Here's how the part is built. I have some questions about the finished solid (model axes, mm). Face numbers are marked on the shaded views. A direction names the side the tool comes from. Round coordinates to 2 decimals unless told otherwise and drop trailing zeros. Write each loop counter-clockwise with the first axis right and the second up, starting at its lowest first coordinate (ties: lowest second). Pieces come first, ordered by that corner, then holes. Notation, with made-up numbers: M 28.25,89 L 67.25,89 A25 ccw 67.25,113 Z; hole C 69.5,32 d8. An arc over 180 degrees is marked long. Use one line per item in the form item = value. Start each with the question number.
Q1. I want a section at A-A on y = -18.5. List the corners of the cut face in (x, z) for me, and give its area (3 significant figures).
Q2. For the marked faces 1, 2 and 3, which set-ups out of +Z, -Z, +X, -X, +Y, -Y let a thin tool reach every point of the face, with its end or its side?
Q3. I want a section at C-C on x = 33. List the corners of the cut face in (y, z) for me, and give its area (3 significant figures).
Q4. I'm going to push flat-ended pins straight in: pin 1 Ø20 at (x, y) = (-30.5, -21.5) entering from +Z; pin 2 Ø7.5 at (y, z) = (-14, 7.5) entering from +X; pin 3 Ø17.5 at (y, z) = (-27.5, -1.5) entering from -X; pin 4 Ø7 at (x, y) = (45, -28.5) entering from +Z. Where does each tip first touch, or does it pass through?
Q5. I want a section at B-B on z = 4. List the corners of the cut face in (x, y) for me.
Q6. I need wall thicknesses on line 1 along X through (y, z) = (-26, -1); line 2 along Z through (x, y) = (49.5, -29.5); line 3 along Z through (x, y) = (-27.5, -25). Which ranges of each line are inside material? Lowest first, please. Write a range as from..to.
```python
from build123d import *

# Parameters (mm, degrees)
F0_W     = 100.000054
F0_H     = 59.99988
F1_DEPTH = 39.99992
F2_W     = 23.5305579296
F2_H     = 25.0000008
F2_W_2   = 25.0000008
F2_H_2   = 34.99993
F3_DEPTH = 40.00092


with BuildPart() as f1:
    # F0 (on Front) → F1 (new body)
    with BuildSketch(Plane.XZ):
        with Locations((3.9102658629, -8.0880385926)):
            Rectangle(F0_W, F0_H)
    extrude(amount=F1_DEPTH)

    # F2 (on face) → F3 (cut, through all)
    with BuildSketch(Plane.XZ.offset(39.99992)):
        with Locations((42.1450138982, 9.4119010074)):
            Rectangle(F2_W, F2_H)
        with Locations((-33.5897607371, 4.4119364074)):
            Rectangle(F2_W_2, F2_H_2)
    extrude(amount=-F3_DEPTH, mode=Mode.SUBTRACT)


solid = f1.part
```
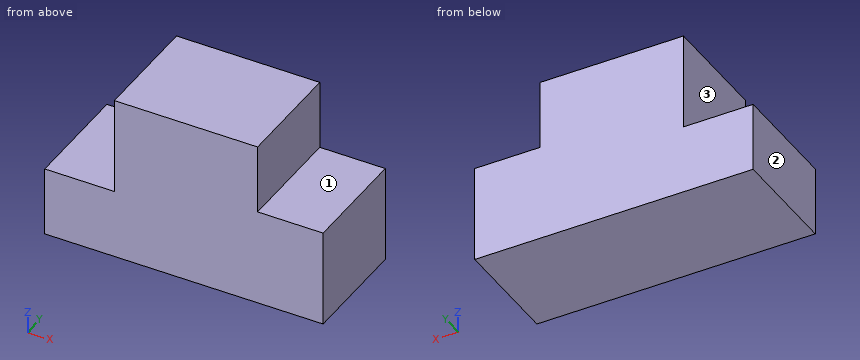
Reported:
q1.outline = M -46.09,-38.09 L 53.91,-38.09 L 53.91,-3.09 L 30.38,-3.09 L 30.38,21.91 L -21.09,21.91 L -21.09,-13.09 L -46.09,-13.09 Z
q1.area = 4,540 mm^2
q2.face_1 = +Z, +X, +Y, -Y
q2.face_2 = +Z, -Z, -X, +Y, -Y
q2.face_3 = +Z, -X, +Y, -Y
q3.outline = M -40,-38.09 L 0,-38.09 L 0,-3.09 L -40,-3.09 Z
q3.area = 1,400 mm^2
q4.pin_1 = 21.91
q4.pin_2 = 30.38
q4.pin_3 = -21.09
q4.pin_4 = -3.09
q5.outline = M -21.09,-40 L 30.38,-40 L 30.38,0 L -21.09,0 Z
q6.line_1 = -21.09..30.38
q6.line_2 = -38.09..-3.09
q6.line_3 = -38.09..-13.09
